```python
from build123d import *

# Parameters (mm, degrees)
F0_W     = 12.7
F0_H     = 279.4
F1_DEPTH = 19.05
F3_D     = 5
F5_D     = 6.8


with BuildPart() as f1:
    # F0 (on Front) → F1 (new body)
    with BuildSketch(Plane.XZ):
        Rectangle(F0_W, F0_H)
    extrude(amount=F1_DEPTH)

    # F3 (through all)
    with Locations(Plane.YZ.offset(6.35)):
        with Locations((-9.525, 127), (-9.525, 63.5), (-9.525, 0), (-9.525, -63.5), (-9.525, -127)):
            Hole(F3_D / 2)

    # F5 (through all)
    with Locations(Plane.XZ.offset(19.05)):
        with Locations((0, 111.125), (0, 79.375), (0, 47.625), (0, 15.875), (0, -15.875), (0, -47.625), (0, -79.375), (0, -111.125)):
            Hole(F5_D / 2)


solid = f1.part
```
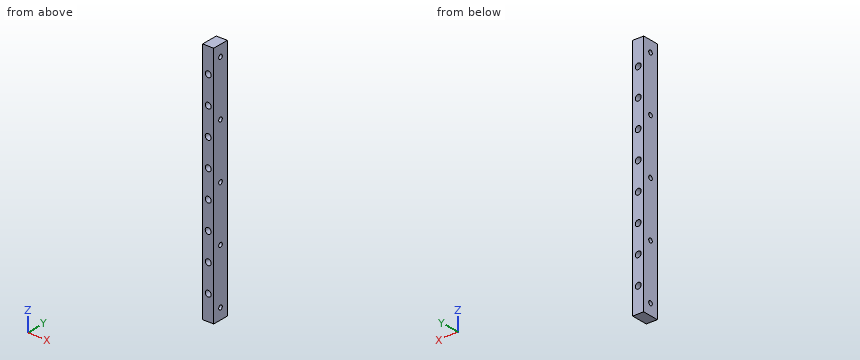
Check sheet for the modelled part. Datum: model origin and axes. Units: mm. Coordinates: 2 decimals unless noted, no trailing zeros. Loops run counter-clockwise (first coordinate to the right, second up) from the corner with the lowest first, then second, coordinate; pieces in that order, holes last.
1) Sectioned sample at A-A (z = 0). Record the boundary of the cut face in (x, y) (3 decimals).
2) Material ranges on probe 1 along Z at (x, y) = (-3.5, -10); probe 2 along Z at (x, y) = (4.75, -7.75); probe 3 along Y at (x, z) = (3, 65.5) (3 decimals), recorded low to high.
3) Gauge pin test, flat end, axial feed: pin 1 (5.5 mm diameter, centred on x = 0, z = 79.375, fed in from +Y). Record the tip position at first contact, or that the pin passes through.
4) Sectioned sample at B-B (x = 0). Count the separate pieces of the cut face and the enclosed holes in it, and give its area (3 significant figures).
Check sheet entries:
1. outline: (-6.35, -19.05) - (6.35, -19.05) - (6.35, -12.025) - (-6.35, -12.025) - close; (-6.35, -7.025) - (6.35, -7.025) - (6.35, 0) - (-6.35, 0) - close
2. probe 1: z = -139.7 to -129.45, -124.55 to -65.95, -61.05 to -2.45, 2.45 to 61.05, 65.95 to 124.55, 129.45 to 139.7
2. probe 2: z = -139.7 to -128.76, -125.24 to -65.26, -61.74 to -1.76, 1.76 to 61.74, 65.26 to 125.24, 128.76 to 139.7
2. probe 3: y = -19.05 to -11.025, -8.025 to 0
3. pin 1: passes through
4. separate pieces: 9
4. enclosed holes: 5
4. area: 4,190 mm2
